Part model, mm, in its own coordinate system. Face numbers are marked on the shaded views. A direction names the side the tool comes from. Round coordinates to 2 decimals unless told otherwise and drop trailing zeros. Loops run counter-clockwise (first coordinate to the right, second up) from the corner with the lowest first, then second, coordinate; pieces in that order, holes last.
1) Mould opens along Y. For the marked faces 1, 2, 3 and 4 say: +Y half, -Y half, draft (parallel to the pull), parting line (faces both ways), or undercut.
2) 3-axis set-ups, long thin cutter, end or side, ignore diameter. For the marked faces 5 and 6: which of +Z, -Z, +X, -X, +Y, -Y reach the whole face in a straight line?
3) Band-saw the part on B-B, the plane z = -31.5. Write the cut outline in (x, y), then the cut area to 3 significant figures.
4) Drop flat-ended pins along their axis: P1, Ø6, axis at x = -3.5, y = -11, coming from the -Z side; P2, Ø12, axis at x = 11, y = -9, coming from the -Z side; P3, Ø2, axis at x = 0, y = 1.5, coming from the -Z side; P4, Ø3, axis at y = -12, z = 21.5, coming from the +X side. Give the stop position or say it passes through.
5) Band-saw the part on C-C, the plane y = -5.75. Write the cut outline in (x, z), then the cut area to 3 significant figures.
6) Probe line 1 (Y direction, x = -13.5, z = -30); line 2 (Z direction, x = -4.5, y = -0.75); line 3 (Z direction, x = -15, y = -3.5). List the from-to ranges inside material, lowest first.
Autodesk Inventor part; units mm, degrees
ref_plane "YZ Plane" through (0, 0, 0) normal (1, 0, 0) x (0, 1, 0)
ref_plane "XZ Plane" through (0, 0, 0) normal (0, 1, 0) x (-1, 0, 0)
ref_plane "XY Plane" through (0, 0, 0) normal (0, 0, 1) x (1, 0, 0)
sketch "Эскиз1" plane through (0, 0, 0) normal (1, 0, 0) x (0, 1, 0)
  line L0 (-15, 100) -> (15, 100)
  line L1 (15, 100) -> (15, -100)
  line L2 (15, -100) -> (-15, -100)
  line L3 (-15, -100) -> (-15, 100)
  line L4 (-21, 0) -> (21, 0) construction
  line L5 (0, -140) -> (0, 140) construction
  point P0 (0, 0)
  dimension "d0" = 200
  dimension "d1" = 30
extrude "Выдавливание2" add sketch "Эскиз1" along normal mid plane 45
fillet "Сопряжение1" radius 15 4 edges at (0, 15, 100) (0, -15, 100) (0, 15, -100) (0, -15, -100)
sketch "Эскиз2" plane through (22.5, 0, 0) normal (1, 0, 0) x (0, 0, -1)
  arc A0 (85, -15) -> (85, 15) centre (85, 0) ccw construction
  line L0 (85, 15) -> (-85, 15) construction
  arc A1 (-85, 15) -> (-85, -15) centre (-85, 0) ccw construction
  line L1 (-85, -15) -> (85, -15) construction
  line L2 (-99, -14) -> (99, -14)
  line L3 (99, -14) -> (99, 14)
  line L4 (99, 14) -> (-99, 14)
  line L5 (-99, 14) -> (-99, -14)
  arc A2 (-85, 14) -> (-99, 0) centre (-85, 0) ccw
  arc A3 (-85, 15) -> (-85, -15) centre (-85, 0) ccw
  arc A4 (-99, 0) -> (-85, -14) centre (-85, 0) ccw
  arc A5 (99, 0) -> (85, 14) centre (85, 0) ccw
  arc A6 (85, -15) -> (85, 15) centre (85, 0) ccw
  arc A7 (85, -14) -> (99, 0) centre (85, 0) ccw
  point P0 (0, 0)
  dimension "d11" = 198
  dimension "d12" = 28
  dimension "d13" = 1
  dimension "d14" = 1
extrude "Выдавливание3" cut sketch "Эскиз2" against normal blind 59 contours A4 A2 L4 A5 A7 L2
properties part number "Лента конвейера"
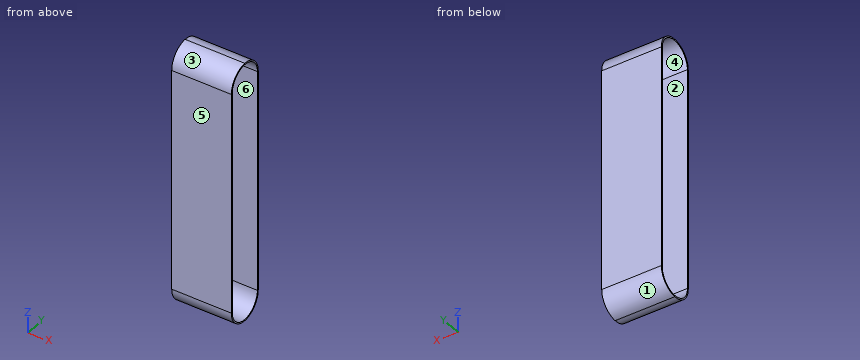
Reported:
1. face 1: +Y half
1. face 2: undercut
1. face 3: -Y half
1. face 4: undercut
2. face 5: +Z, -Z, +X, -X, -Y
2. face 6: +X, -X
3. outline: (-22.5, -15) - (22.5, -15) - (22.5, -14) - (-22.5, -14) - close; (-22.5, 14) - (22.5, 14) - (22.5, 15) - (-22.5, 15) - close
3. area: 90.0 mm2
4. P1: stops at z = -97.69
4. P2: stops at z = -99.7
4. P3: stops at z = -99.99
4. P4: passes through
5. outline: (-22.5, -98.85) - (22.5, -98.85) - (22.5, -97.76) - (-22.5, -97.76) - close; (-22.5, 97.76) - (22.5, 97.76) - (22.5, 98.85) - (-22.5, 98.85) - close
5. area: 98.1 mm2
6. line 1: y = -15 to -14, 14 to 15
6. line 2: z = -99.98 to -98.98, 98.98 to 99.98
6. line 3: z = -99.59 to -98.56, 98.56 to 99.59
